```python
from build123d import *

# Parameters (mm, degrees)
ESTRUSIONE_ESTRUSIONE1_DEPTH = 5
SCHIZZO2_W                   = 73
SCHIZZO2_H                   = 5
ESTRUSIONE_ESTRUSIONE2_DEPTH = 53
SCHIZZO4_R                   = 1.25
TAGLIO_ESTRUSIONE1_DEPTH     = 10
SCHIZZO1_3_W                 = 3.5
SCHIZZO1_3_H                 = 11
ESTRUSIONE_ESTRUSIONE3_DEPTH = 44
SCHIZZO5_R                   = 1.625
TAGLIO_ESTRUSIONE2_DEPTH     = 91
SCHIZZO2_3_W                 = 90
SCHIZZO2_3_H                 = 5
ESTRUSIONE_ESTRUSIONE4_DEPTH = 52
SCHIZZO8_R                   = 1.75
TAGLIO_ESTRUSIONE3_DEPTH     = 6
ESTRUSIONE_ESTRUSIONE5_DEPTH = 11
ESTRUSIONE_ESTRUSIONE6_DEPTH = 5


with BuildPart() as part:
    # Schizzo1 → Estrusione-Estrusione1 (new body)
    with BuildSketch(Plane(origin=(0, 0, 0), x_dir=(1, 0, 0), z_dir=(0, 1, 0))):
        Polygon((45, 10), (36.5, 10), (36.5, 35), (-36.5, 35), (-36.5, 10), (-45, 10), (-45, 6), (-41.5, 6), (-41.5, -5), (-45, -5), (-45, -35), (45, -35), (45, -5), (41.5, -5), (41.5, 6), (45, 6), align=None)
    extrude(amount=ESTRUSIONE_ESTRUSIONE1_DEPTH)

    # Schizzo2 → Estrusione-Estrusione2 (add)
    with BuildSketch(Plane(origin=(0, 5, 0), x_dir=(1, 0, 0), z_dir=(0, 1, 0))):
        with Locations((0, 32.5)):
            Rectangle(SCHIZZO2_W, SCHIZZO2_H)
    extrude(amount=ESTRUSIONE_ESTRUSIONE2_DEPTH)

    # Schizzo4 → Taglio-Estrusione1 (cut)
    with BuildSketch(Plane(origin=(0, 0, -35), x_dir=(-1, 0, 0), z_dir=(0, 0, -1))):
        with Locations((-33, 54.5)):
            Circle(SCHIZZO4_R)
        with Locations((33, 54.5)):
            Circle(SCHIZZO4_R)
        with Locations((33, 8.5)):
            Circle(SCHIZZO4_R)
        with Locations((-33, 8.5)):
            Circle(SCHIZZO4_R)
    extrude(amount=-TAGLIO_ESTRUSIONE1_DEPTH, mode=Mode.SUBTRACT)

    # Schizzo1_3 → Estrusione-Estrusione3 (add)
    with BuildSketch(Plane(origin=(0, 0, 0), x_dir=(1, 0, 0), z_dir=(0, 1, 0))):
        with Locations((-43.25, 0.5)):
            Rectangle(SCHIZZO1_3_W, SCHIZZO1_3_H)
        with Locations((43.25, 0.5)):
            Rectangle(SCHIZZO1_3_W, SCHIZZO1_3_H)
    extrude(amount=ESTRUSIONE_ESTRUSIONE3_DEPTH)

    # Schizzo5 → Taglio-Estrusione2 (cut, through all)
    with BuildSketch(Plane.ZY.offset(45)):
        with Locations((-0.5, 40.5)):
            Circle(SCHIZZO5_R)
        with Locations((-0.5, 23.5)):
            Circle(SCHIZZO5_R)
    extrude(amount=-TAGLIO_ESTRUSIONE2_DEPTH, mode=Mode.SUBTRACT)

    # Schizzo2_3 → Estrusione-Estrusione4 (add)
    with BuildSketch(Plane(origin=(0, 5, 0), x_dir=(1, 0, 0), z_dir=(0, 1, 0))):
        with Locations((0, -32.5)):
            Rectangle(SCHIZZO2_3_W, SCHIZZO2_3_H)
    extrude(amount=ESTRUSIONE_ESTRUSIONE4_DEPTH)

    # Schizzo8 → Taglio-Estrusione3 (cut, through all)
    with BuildSketch(Plane(origin=(0, 0, 30), x_dir=(-1, 0, 0), z_dir=(0, 0, -1))):
        with Locations((-39, 31)):
            Circle(SCHIZZO8_R)
        with Locations((39, 31)):
            Circle(SCHIZZO8_R)
    extrude(amount=-TAGLIO_ESTRUSIONE3_DEPTH, mode=Mode.SUBTRACT)

    # Schizzo11 → Estrusione-Estrusione5 (add)
    with BuildSketch(Plane.XY.offset(5)):
        Polygon((41.5, 17.747952022), (26.515389788, 5), (41.5, 5), align=None)
        Polygon((-26.515389788, 5), (-41.5, 5), (-41.5, 17.747952022), align=None)
    extrude(amount=-ESTRUSIONE_ESTRUSIONE5_DEPTH)

    # Schizzo13 → Estrusione-Estrusione6 (add, symmetric)
    with BuildSketch(Plane.ZY.offset(16.5)):
        Polygon((-30, 25), (-20, 5), (-30, 5), align=None)
    estrusione_estrusione6 = extrude(amount=ESTRUSIONE_ESTRUSIONE6_DEPTH, both=True)

    # Specchia1: Estrusione-Estrusione6 across plane
    add(estrusione_estrusione6.mirror(Plane(origin=(0, 0, 0), x_dir=(0, 0, 1), z_dir=(1, 0, 0))))


solid = part.part
```
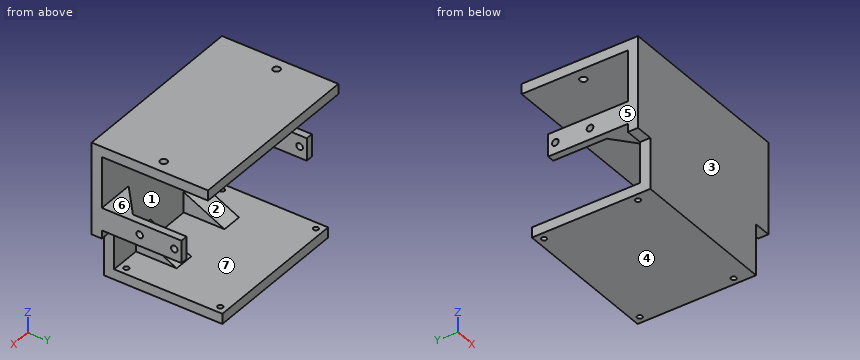
The listing builds one solid part. Answer for the finished solid, in the listing's coordinates (mm). Face numbers are marked on the shaded views. A direction names the side the tool comes from. Give positions to 0.01 mm unless a question says otherwise; leave off trailing zeros. Order: outer loops, then holes, each group sorted by start corner. A loop starts at its lowest first (then second) coordinate and runs counter-clockwise, first axis right, second up. Notation, with made-up numbers: (87, 47.5) -> (125, 47.5) arc R18 ccw to (125, 58.5) -> close; hole circle Ø2 at (66, -38.75). An arc over 180 degrees is marked (long way). One line per item, written item: value.
1) Find section D-D, the plane z = -23. Determine the outline of the cut face in (x, y).
Reported:
outline: (-36.5, 0) -> (36.5, 0) -> (36.5, 5) -> (21.5, 5) -> (21.5, 11) -> (11.5, 11) -> (11.5, 5) -> (-11.5, 5) -> (-11.5, 11) -> (-21.5, 11) -> (-21.5, 5) -> (-36.5, 5) -> close
2) Flat-ended cylindrical pins translate along their axes: P1, Ø12, axis at y = 18, z = -21, coming from the -X side; P2, Ø12, axis at y = 7, z = -21, coming from the -X side; P3, Ø4, axis at x = 43, z = 2, coming from the +Y side. Find the tip coordinate at first contact, or state that the pin passes through.
Reported:
P1: stops at x = -21.5
P2: stops at x = -36.5
P3: stops at y = 44
3) A tool of negligible diameter and unlimited length cuts with its end or side. For the marked faces 5, 6 and 7, from which of +Z, -Z, +X, -X, +Y, -Y can it reach the whole face along a straight path? Write none if from no direction.
Reported:
face 5: +Z, -Z, -X, +Y, -Y
face 6: +X, -X, +Y
face 7: +Y
4) Find the intervals of material crossed by line 1 (Y direction, x = 33, z = -33); line 2 (Y direction, x = 43.05, z = -0.5) (3 decimals); line 3 (X direction, y = 33.5, z = -0.5), in increasing order.
Reported:
line 1: y = 0 to 7.25, 9.75 to 53.25, 55.75 to 58
line 2: y = 0 to 21.875, 25.125 to 38.875, 42.125 to 44
line 3: x = -45 to -41.5, 41.5 to 45
5) Find section B-B, the plane z = -0.5. Determine the outline of the cut face in (x, y) (3 decimals).
Reported:
outline: (-45, 0) -> (45, 0) -> (45, 21.875) -> (41.5, 21.875) -> (41.5, 17.748) -> (26.515, 5) -> (-26.515, 5) -> (-41.5, 17.748) -> (-41.5, 21.875) -> (-45, 21.875) -> close; (-45, 25.125) -> (-41.5, 25.125) -> (-41.5, 38.875) -> (-45, 38.875) -> close; (-45, 42.125) -> (-41.5, 42.125) -> (-41.5, 44) -> (-45, 44) -> close; (41.5, 25.125) -> (45, 25.125) -> (45, 38.875) -> (41.5, 38.875) -> close; (41.5, 42.125) -> (45, 42.125) -> (45, 44) -> (41.5, 44) -> close
6) Find section C-C, the plane y = 54.5. Determine the outline of the cut face in (x, z).
Reported:
outline: (-45, 30) -> (45, 30) -> (45, 35) -> (-45, 35) -> close; (-36.5, -35) -> (-34.25, -35) -> (-34.25, -30) -> (-36.5, -30) -> close; (-31.75, -35) -> (31.75, -35) -> (31.75, -30) -> (-31.75, -30) -> close; (34.25, -35) -> (36.5, -35) -> (36.5, -30) -> (34.25, -30) -> close
7) Determine the mould class of the marked faces 1, 2, 3 and 4 for opening direction Z: pulls with the +Z half, pulls with the -Z half, needs draft (parallel to the pull), parting line crosses it, or undercut.
Reported:
face 1: undercut
face 2: undercut
face 3: needs draft
face 4: pulls with the -Z half
8) Find section A-A, the plane y = 23.5. Count the separate pieces of the cut face and the enclosed holes in it, plus the area to 3 significant figures.
Reported:
separate pieces: 6
enclosed holes: 0
area: 884 mm^2
